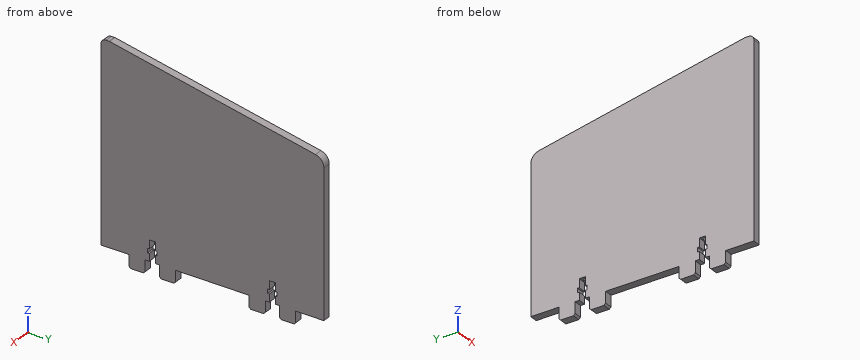
```python
from build123d import *

# Parameters (mm, degrees)
EXTRUDE1_DEPTH = 4.6
SKETCH2_R      = 1
EXTRUDE2_DEPTH = 1


with BuildPart() as part:
    # Sketch1 → Extrude1 (new body)
    with BuildSketch(Plane(origin=(0, 0, 0), x_dir=(0, 0, -1), z_dir=(1, 0, 0))):
        with BuildLine():
            Line((120.06791936, 91.267546052), (126.56791936, 91.267546052))
            Line((126.56791936, 91.267546052), (127.56791936, 92.267546052))
            Line((127.56791936, 92.267546052), (127.56791936, 99.767546052))
            Line((127.56791936, 99.767546052), (126.56791936, 100.767546052))
            Line((126.56791936, 100.767546052), (120.06791936, 100.767546052))
            Line((120.06791936, 100.767546052), (120.06791936, 103.142546052))
            Line((120.06791936, 103.142546052), (115.56791936, 103.142546052))
            Line((115.56791936, 103.142546052), (115.56791936, 102.142546052))
            Line((115.56791936, 102.142546052), (113.06791936, 102.142546052))
            Line((113.06791936, 102.142546052), (113.06791936, 103.142546052))
            Line((113.06791936, 103.142546052), (108.06791936, 103.142546052))
            Line((108.06791936, 103.142546052), (108.06791936, 106.642546052))
            Line((108.06791936, 106.642546052), (113.06791936, 106.642546052))
            Line((113.06791936, 106.642546052), (113.06791936, 107.642546052))
            Line((113.06791936, 107.642546052), (115.56791936, 107.642546052))
            Line((115.56791936, 107.642546052), (115.56791936, 106.642546052))
            Line((115.56791936, 106.642546052), (120.06791936, 106.642546052))
            Line((120.06791936, 106.642546052), (120.06791936, 109.017546052))
            Line((120.06791936, 109.017546052), (126.56791936, 109.017546052))
            Line((126.56791936, 109.017546052), (127.56791936, 110.017546052))
            Line((127.56791936, 110.017546052), (127.56791936, 117.517546052))
            Line((127.56791936, 117.517546052), (126.56791936, 118.517546052))
            Line((126.56791936, 118.517546052), (120.06791936, 118.517546052))
            Line((120.06791936, 118.517546052), (120.06791936, 134.892546052))
            Line((120.06791936, 134.892546052), (34.986742776, 134.892546052))
            ThreePointArc((34.986742776, 134.892546052), (31.182809342, 133.5325989), (29.103258722, 130.069242862))
            Line((29.103258722, 130.069242862), (5.087338684, 9.989642673))
            ThreePointArc((5.087338684, 9.989642673), (5.072786033, 9.892064156), (5.06791936, 9.793526538))
            Line((5.06791936, 9.793526538), (5.06791936, 7.892546052))
            ThreePointArc((5.06791936, 7.892546052), (5.946599016, 5.771225708), (8.06791936, 4.892546052))
            Line((8.06791936, 4.892546052), (120.06791936, 4.892546052))
            Line((120.06791936, 4.892546052), (120.06791936, 21.267546052))
            Line((120.06791936, 21.267546052), (126.56791936, 21.267546052))
            Line((126.56791936, 21.267546052), (127.56791936, 22.267546052))
            Line((127.56791936, 22.267546052), (127.56791936, 29.767546052))
            Line((127.56791936, 29.767546052), (126.56791936, 30.767546052))
            Line((126.56791936, 30.767546052), (120.06791936, 30.767546052))
            Line((120.06791936, 30.767546052), (120.06791936, 33.142546052))
            Line((120.06791936, 33.142546052), (115.56791936, 33.142546052))
            Line((115.56791936, 33.142546052), (115.56791936, 32.142546052))
            Line((115.56791936, 32.142546052), (113.06791936, 32.142546052))
            Line((113.06791936, 32.142546052), (113.06791936, 33.142546052))
            Line((113.06791936, 33.142546052), (108.06791936, 33.142546052))
            Line((108.06791936, 33.142546052), (108.06791936, 36.642546052))
            Line((108.06791936, 36.642546052), (113.06791936, 36.642546052))
            Line((113.06791936, 36.642546052), (113.06791936, 37.642546052))
            Line((113.06791936, 37.642546052), (115.56791936, 37.642546052))
            Line((115.56791936, 37.642546052), (115.56791936, 36.642546052))
            Line((115.56791936, 36.642546052), (120.06791936, 36.642546052))
            Line((120.06791936, 36.642546052), (120.06791936, 39.017546052))
            Line((120.06791936, 39.017546052), (126.56791936, 39.017546052))
            Line((126.56791936, 39.017546052), (127.56791936, 40.017546052))
            Line((127.56791936, 40.017546052), (127.56791936, 47.517546052))
            Line((127.56791936, 47.517546052), (126.56791936, 48.517546052))
            Line((126.56791936, 48.517546052), (120.06791936, 48.517546052))
            Line((120.06791936, 48.517546052), (120.06791936, 91.267546052))
        make_face()
    extrude(amount=EXTRUDE1_DEPTH)

    # Sketch2 → Extrude2 (cut)
    with BuildSketch(Plane(origin=(0, 0, -108.06791936), x_dir=(-1, 0, 0), z_dir=(0, 0, -1))):
        with Locations((-2.3, 34.892546052)):
            Circle(SKETCH2_R)
        with Locations((-2.3, 104.892546052)):
            Circle(SKETCH2_R)
    extrude(amount=-EXTRUDE2_DEPTH, mode=Mode.SUBTRACT)


solid = part.part
```
Source: CAD feature listing. Evaluate the final solid. Frame: model axes, mm. Coordinates: 2 decimals unless noted, no trailing zeros. Write each loop counter-clockwise with the first axis right and the second up, starting at its lowest first coordinate (ties: lowest second). Pieces come first, ordered by that corner, then holes. Notation, with made-up numbers: M 23.25,-25.5 L 49.25,-25.5 A23 cw 49.25,12.5 Z; hole C 64,37 d4. An arc over 180 degrees is marked long. Answer as a JSON object with one key per item and string values.
1. Ray query, L1, parallel to Y at x = 2.3, z = -107.55; L2, parallel to Y at x = 0.8, z = -121.5; L3, parallel to Y at x = 0.65, z = -112. Return the intervals inside material, ascending.
Evaluation:
{"L1": "4.89 to 33.89, 35.89 to 103.89, 105.89 to 134.89", "L2": "21.27 to 30.77, 39.02 to 48.52, 91.27 to 100.77, 109.02 to 118.52", "L3": "4.89 to 33.14, 36.64 to 103.14, 106.64 to 134.89"}
2. Cut plane A-A on y = 44.5. Output: boundary loops of the cut face in (x, z).
Evaluation:
{"outline": "M 0,-127.57 L 4.6,-127.57 L 4.6,-11.99 L 0,-11.99 Z"}
3. Cut plane B-B on y = 89. Output: boundary loops of the cut face in (x, z), plus the area to 3 significant figures.
Evaluation:
{"outline": "M 0,-120.07 L 4.6,-120.07 L 4.6,-20.89 L 0,-20.89 Z", "area": "456 mm^2"}
4. Contact query for flat-ended pins moving along their axis: P1, Ø2.5, axis at x = 2.5, z = -125, coming from the +Y side; P2, Ø2, axis at x = 2, y = 90.5, coming from the +Z side; P3, Ø1.1, axis at x = 1.5, y = 107.5, coming from the +Z side. Output: stop coordinate, or through.
Evaluation:
{"P1": "y = 118.52", "P2": "z = -20.99", "P3": "z = -24.48"}
